from build123d import *

# Parameters (mm, degrees)
BOSS_EXTRUDE1_DEPTH = 5
SHELL1_T            = -2
FILLET1_R           = 1
SKETCH2_R           = 13.5
BOSS_EXTRUDE2_DEPTH = 3


with BuildPart() as part:
    # Sketch1 → Boss-Extrude1 (new body)
    with BuildSketch(Plane(origin=(0, 0, 0), x_dir=(1, 0, 0), z_dir=(0, 1, 0))):
        with BuildLine():
            Line((-15, -18), (15, -18))
            ThreePointArc((15, -18), (17.121320344, -17.121320344), (18, -15))
            Line((18, -15), (18, 15))
            ThreePointArc((18, 15), (17.121320344, 17.121320344), (15, 18))
            Line((15, 18), (-15, 18))
            ThreePointArc((-15, 18), (-17.121320344, 17.121320344), (-18, 15))
            Line((-18, 15), (-18, -15))
            ThreePointArc((-18, -15), (-17.121320344, -17.121320344), (-15, -18))
        make_face()
    extrude(amount=BOSS_EXTRUDE1_DEPTH)

    # Shell1
    shell1_openings = [part.faces().sort_by_distance(p)[0] for p in [
        (0, 0, 0),
    ]]
    offset(amount=SHELL1_T, openings=shell1_openings, kind=Kind.INTERSECTION)

    # Fillet1
    fillet1_edges = [part.edges().sort_by_distance(p)[0] for p in [
        (17.121320344, 5, 17.121320344),
        (18, 5, 0),
        (17.121320344, 5, -17.121320344),
        (0, 5, -18),
        (-17.121320344, 5, -17.121320344),
        (-18, 5, 0),
        (-17.121320344, 5, 17.121320344),
        (0, 5, 18),
    ]]
    fillet(fillet1_edges, radius=FILLET1_R)

    # Sketch2 → Boss-Extrude2 (add)
    with BuildSketch(Plane.XZ.offset(-3)):
        with Locations(Location((0, 0, 0), (0, 0, 270))):
            Circle(SKETCH2_R)
    extrude(amount=BOSS_EXTRUDE2_DEPTH)


solid = part.part
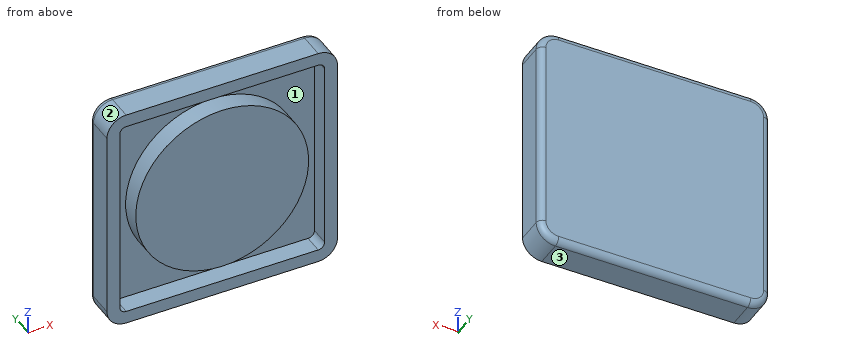
Can you work these out from the model? Positions are in its coordinate system, mm. Face numbers are marked on the shaded views. Coordinates: 2 decimals unless noted, no trailing zeros. Loops run counter-clockwise (first coordinate to the right, second up) from the corner with the lowest first, then second, coordinate; pieces in that order, holes last. Notation, with made-up numbers: M 37,-18.75 L 70,-18.75 A22 cw 70,7.25 Z; hole C 16.25,78 d8. An arc over 180 degrees is marked long. Return JSON: item names as keys, results as strings. Group by question number.
Item 1: Thinking about a two-plate mould opening in X: for the marked faces 1, 2 and 3, which applies, released by +X, released by -X, zero draft, split by the parting line, or undercut?
Item 2: If I drill on L1, parallel to X at y = 1.4, z = 11; L2, parallel to Z at x = -1.5, y = 1.9; L3, parallel to X at y = 1.65, z = 8, over which ranges is the centre line in solid material (lowest first)? Write a range as from..to.
Item 3: Imagine slicing it at A-A (z = 0). Please give me the cut outline in (x, y), and give its area (3 significant figures).
Item 4: Imagine slicing it at C-C (y = 4.5). Please give me the cut outline in (x, z).
Item 5: Imagine slicing it at B-B (x = 0). Please give me the cut outline in (y, z), and give its area (3 significant figures).
Verdict:
{
 "1": {"face 1": "undercut", "face 2": "released by -X", "face 3": "zero draft"},
 "2": {"L1": "x = -18..-16, -7.83..7.83, 16..18", "L2": "z = -18..-16, -13.42..13.42, 16..18", "L3": "x = -18..-16, -10.87..10.87, 16..18"},
 "3": {"outline": "M -18,0 L -16,0 L -16,3 L -13.5,3 L -13.5,0 L 13.5,0 L 13.5,3 L 16,3 L 16,0 L 18,0 L 18,4 A1 ccw 17,5 L -17,5 A1 ccw -18,4 Z", "area": "165 mm^2"},
 "4": {"outline": "M -17.87,-15 A2.87 ccw -15,-17.87 L 15,-17.87 A2.87 ccw 17.87,-15 L 17.87,15 A2.87 ccw 15,17.87 L -15,17.87 A2.87 ccw -17.87,15 Z"},
 "5": {"outline": "M 0,-18 L 4,-18 A1 ccw 5,-17 L 5,17 A1 ccw 4,18 L 0,18 L 0,16 L 3,16 L 3,13.5 L 0,13.5 L 0,-13.5 L 3,-13.5 L 3,-16 L 0,-16 Z", "area": "165 mm^2"}
}
